The listing builds one solid part. Answer for the finished solid, in the listing's coordinates (mm). A direction names the side the tool comes from. Round coordinates to 2 decimals unless told otherwise and drop trailing zeros. Loops run counter-clockwise (first coordinate to the right, second up) from the corner with the lowest first, then second, coordinate; pieces in that order, holes last. Notation, with made-up numbers: M 79.25,49.5 L 93.25,49.5 A33 ccw 93.25,79.5 Z; hole C 34,20 d2. An arc over 180 degrees is marked long. Answer as a JSON object with one key per item and string values.
```python
from build123d import *

# Parameters (mm, degrees)
F3_DEPTH = 36.581717


with BuildPart() as f1:
    # F0 (on Right) → F1 (revolve)
    with BuildSketch(Plane.YZ):
        Polygon((-12.7, 0), (0, 0), (0, 50.8), (-12.7, 50.8), (-12.7, 47.625), (-9.525, 44.960859), (-10.795, 44.960859), (-10.795, 43.690859), (-9.525, 43.690859), (-9.525, 7.109141), (-10.795, 7.109141), (-10.795, 5.839141), (-9.525, 5.839141), (-12.7, 3.175), align=None)
    revolve(axis=Axis((0, 0, 25.4), (0, 0, -1)))

    # F2 (on face) → F3 (cut, through all)
    with BuildSketch(Plane.XY.offset(7.109141)):
        with BuildLine():
            Line((3.159052, -7.626626), (3.64506, -8.799953))
            ThreePointArc((3.64506, -8.799953), (4.490054, -8.4003), (5.291806, -7.919748))
            Line((5.291806, -7.919748), (4.586232, -6.863782))
            ThreePointArc((4.586232, -6.863782), (3.89138, -7.28026), (3.159052, -7.626626))
        make_face()
        with BuildLine():
            Line((0, -8.255), (0, -9.525))
            ThreePointArc((0, -9.525), (0.933613, -9.479135), (1.858235, -9.34198))
            Line((1.858235, -9.34198), (1.610471, -8.096382))
            ThreePointArc((1.610471, -8.096382), (0.809131, -8.21525), (0, -8.255))
        make_face()
        with BuildLine():
            ThreePointArc((6.863782, -4.586232), (6.381201, -5.236917), (5.837166, -5.837166))
            Line((5.837166, -5.837166), (6.735192, -6.735192))
            ThreePointArc((6.735192, -6.735192), (7.362925, -6.042596), (7.919748, -5.291806))
            Line((7.919748, -5.291806), (6.863782, -4.586232))
        make_face()
        with BuildLine():
            ThreePointArc((8.096382, -1.610471), (7.899542, -2.3963), (7.626626, -3.159052))
            Line((7.626626, -3.159052), (8.799953, -3.64506))
            ThreePointArc((8.799953, -3.64506), (9.114857, -2.764962), (9.34198, -1.858235))
            Line((9.34198, -1.858235), (8.096382, -1.610471))
        make_face()
        with BuildLine():
            Line((-7.626626, -3.159052), (-8.799953, -3.64506))
            ThreePointArc((-8.799953, -3.64506), (-8.4003, -4.490054), (-7.919748, -5.291806))
            Line((-7.919748, -5.291806), (-6.863782, -4.586232))
            ThreePointArc((-6.863782, -4.586232), (-7.28026, -3.89138), (-7.626626, -3.159052))
        make_face()
        with BuildLine():
            Line((-8.255, 0), (-9.525, 0))
            ThreePointArc((-9.525, 0), (-9.479135, -0.933613), (-9.34198, -1.858235))
            Line((-9.34198, -1.858235), (-8.096382, -1.610471))
            ThreePointArc((-8.096382, -1.610471), (-8.21525, -0.809131), (-8.255, 0))
        make_face()
        with BuildLine():
            Line((-5.291806, -7.919748), (-4.586232, -6.863782))
            ThreePointArc((-4.586232, -6.863782), (-5.236917, -6.381201), (-5.837166, -5.837166))
            Line((-5.837166, -5.837166), (-6.735192, -6.735192))
            ThreePointArc((-6.735192, -6.735192), (-6.042596, -7.362925), (-5.291806, -7.919748))
        make_face()
        with BuildLine():
            Line((-3.159052, -7.626626), (-3.64506, -8.799953))
            ThreePointArc((-3.64506, -8.799953), (-2.764962, -9.114857), (-1.858235, -9.34198))
            Line((-1.858235, -9.34198), (-1.610471, -8.096382))
            ThreePointArc((-1.610471, -8.096382), (-2.3963, -7.899542), (-3.159052, -7.626626))
        make_face()
        with BuildLine():
            Line((-3.159052, 7.626626), (-3.64506, 8.799953))
            ThreePointArc((-3.64506, 8.799953), (-4.490054, 8.4003), (-5.291806, 7.919748))
            Line((-5.291806, 7.919748), (-4.586232, 6.863782))
            ThreePointArc((-4.586232, 6.863782), (-3.89138, 7.28026), (-3.159052, 7.626626))
        make_face()
        with BuildLine():
            Line((0, 8.255), (0, 9.525))
            ThreePointArc((0, 9.525), (-0.933613, 9.479135), (-1.858235, 9.34198))
            Line((-1.858235, 9.34198), (-1.610471, 8.096382))
            ThreePointArc((-1.610471, 8.096382), (-0.809131, 8.21525), (0, 8.255))
        make_face()
        with BuildLine():
            Line((-7.919748, 5.291806), (-6.863782, 4.586232))
            ThreePointArc((-6.863782, 4.586232), (-6.381201, 5.236917), (-5.837166, 5.837166))
            Line((-5.837166, 5.837166), (-6.735192, 6.735192))
            ThreePointArc((-6.735192, 6.735192), (-7.362925, 6.042596), (-7.919748, 5.291806))
        make_face()
        with BuildLine():
            Line((-7.626626, 3.159052), (-8.799953, 3.64506))
            ThreePointArc((-8.799953, 3.64506), (-9.114857, 2.764962), (-9.34198, 1.858235))
            Line((-9.34198, 1.858235), (-8.096382, 1.610471))
            ThreePointArc((-8.096382, 1.610471), (-7.899542, 2.3963), (-7.626626, 3.159052))
        make_face()
        with BuildLine():
            Line((7.626626, 3.159052), (8.799953, 3.64506))
            ThreePointArc((8.799953, 3.64506), (8.4003, 4.490054), (7.919748, 5.291806))
            Line((7.919748, 5.291806), (6.863782, 4.586232))
            ThreePointArc((6.863782, 4.586232), (7.28026, 3.89138), (7.626626, 3.159052))
        make_face()
        with BuildLine():
            Line((8.255, 0), (9.525, 0))
            ThreePointArc((9.525, 0), (9.479135, 0.933613), (9.34198, 1.858235))
            Line((9.34198, 1.858235), (8.096382, 1.610471))
            ThreePointArc((8.096382, 1.610471), (8.21525, 0.809131), (8.255, 0))
        make_face()
        with BuildLine():
            Line((5.291806, 7.919748), (4.586232, 6.863782))
            ThreePointArc((4.586232, 6.863782), (5.236917, 6.381201), (5.837166, 5.837166))
            Line((5.837166, 5.837166), (6.735192, 6.735192))
            ThreePointArc((6.735192, 6.735192), (6.042596, 7.362925), (5.291806, 7.919748))
        make_face()
        with BuildLine():
            Line((3.159052, 7.626626), (3.64506, 8.799953))
            ThreePointArc((3.64506, 8.799953), (2.764962, 9.114857), (1.858235, 9.34198))
            Line((1.858235, 9.34198), (1.610471, 8.096382))
            ThreePointArc((1.610471, 8.096382), (2.3963, 7.899542), (3.159052, 7.626626))
        make_face()
    extrude(amount=F3_DEPTH, mode=Mode.SUBTRACT)


solid = f1.part
```
Item 1: The part is cut by section A-A (z = 5). Give the vertices of the cut face in (x, y), then the cut area to 3 significant figures.
Values follow:
{"outline": "C 0,0 d21.05", "area": "348 mm^2"}
Item 2: Which of the six approach directions +Z, -Z, +X, -X, +Y, -Y give full straight-line access (tool end or side, diameter ignored) to faces 5 (the face through (-1, 9, 43.691)), 6 (the face through (1, -9, 43.691)), 7 (the face through (-7, 6, 43.691))?
Values follow:
{"face 5": "+Y", "face 6": "-Y", "face 7": "none"}
Item 3: Straight lines are drawn through the part: line 1 (Z direction, x = 0.75, y = -9); line 2 (Z direction, x = -9.25, y = -4.75); line 3 (Y direction, x = -0.25, z = 12). For each, find the intervals that lie inside material, in ascending order.
Values follow:
{"line 1": "0 to 7.11, 43.69 to 50.8", "line 2": "0 to 5.11, 5.84 to 7.11, 43.69 to 44.96, 45.69 to 50.8", "line 3": "-9.52 to 8.25"}
Item 4: Flat-ended cylindrical pins translate along their axes: P1, Ø1.5, axis at x = 5.5, z = 29.5, coming from the -Y side; P2, Ø5, axis at x = 3, z = 10, coming from the +Y side; P3, Ø1.4, axis at x = -8.5, z = 29, coming from the -Y side. Find the tip coordinate at first contact, or state that the pin passes through.
Values follow:
{"P1": "y = -7.92", "P2": "y = 9.51", "P3": "y = -5.47"}
Item 5: Determine the mould class of faces 1 (the face through (-7.296, 7.956, 44.317)), 2 (the face through (-5.228, -6.388, 25.144)), 3 (the face through (8.214, 0.82, 25.144)), 4 (the face through (0, -9, 25)) for opening direction Y: released by +Y, released by -Y, zero draft, split by the parting line, or undercut.
Values follow:
{"face 1": "split by the parting line", "face 2": "undercut", "face 3": "undercut", "face 4": "zero draft"}
